Check sheet for the modelled part. Datum: model origin and axes. Units: mm. Round coordinates to 2 decimals unless told otherwise and drop trailing zeros. Order: outer loops, then holes, each group sorted by start corner. A loop starts at its lowest first (then second) coordinate and runs counter-clockwise, first axis right, second up. Notation, with made-up numbers: (-14, -8.5) -> (44, -8.5) arc R18 ccw to (44, 2.5) -> close; hole circle Ø1 at (67.5, 55.5). An arc over 180 degrees is marked (long way). Answer in a Markdown table with one row per item.
```python
from build123d import *

# Parameters (mm, degrees)
SKETCH_1_W          = 164
SKETCH_1_H          = 215
SKETCH_1_R          = 14.5
EXTRUDE_1_DEPTH     = 3
SKETCH_2_R          = 2
CUT_EXTRUDE_1_DEPTH = 3
SKETCH_3_W          = 3
SKETCH_3_H          = 25
CUT_EXTRUDE_2_DEPTH = 10
SKETCH_4_W          = 15
SKETCH_4_H          = 3
CUT_EXTRUDE_3_DEPTH = 10
SKETCH_6_W          = 10
SKETCH_6_H          = 190
EXTRUDE_2_DEPTH     = 3
CHAMFER_1_SIZE      = 25
CHAMFER_1_SIZE_2    = 14.43375673
FILLET_3_R          = 20
FILLET_4_R          = 10


with BuildPart() as part:
    # 草图1 → 凸台-拉伸1 (new body)
    with BuildSketch(Plane(origin=(0, 0, 0), x_dir=(1, 0, 0), z_dir=(0, 1, 0))):
        with Locations((47, 70)):
            Rectangle(SKETCH_1_W, SKETCH_1_H)
        with Locations(Location((94, 40, 0), (0, 0, 270))):
            Circle(SKETCH_1_R, mode=Mode.SUBTRACT)
        with Locations(Location((0, 40, 0), (0, 0, 270))):
            Circle(SKETCH_1_R, mode=Mode.SUBTRACT)
        with Locations(Location((0, 145, 0), (0, 0, 270))):
            Circle(SKETCH_1_R, mode=Mode.SUBTRACT)
        with Locations(Location((94, 145, 0), (0, 0, 270))):
            Circle(SKETCH_1_R, mode=Mode.SUBTRACT)
    extrude(amount=EXTRUDE_1_DEPTH)

    # 草图2 → 切除-拉伸1 (cut)
    with BuildSketch(Plane(origin=(0, 3, 0), x_dir=(1, 0, 0), z_dir=(0, 1, 0))):
        with Locations(Location((0, -27.5, 0), (0, 0, 270))):
            Circle(SKETCH_2_R)
        with Locations(Location((-15, -27.5, 0), (0, 0, 270))):
            Circle(SKETCH_2_R)
        with Locations(Location((15, -27.5, 0), (0, 0, 90))):
            Circle(SKETCH_2_R)
        with Locations(Location((79, -27.5, 0), (0, 0, 270))):
            Circle(SKETCH_2_R)
        with Locations(Location((109, -27.5, 0), (0, 0, 90))):
            Circle(SKETCH_2_R)
        with Locations(Location((94, -27.5, 0), (0, 0, 90))):
            Circle(SKETCH_2_R)
    extrude(amount=-CUT_EXTRUDE_1_DEPTH, mode=Mode.SUBTRACT)

    # 草图3 → 切除-拉伸2 (cut)
    with BuildSketch(Plane(origin=(0, 3, 0), x_dir=(1, 0, 0), z_dir=(0, 1, 0))):
        with Locations((28.5, 135)):
            Rectangle(SKETCH_3_W, SKETCH_3_H)
        with Locations((65.5, 135)):
            Rectangle(SKETCH_3_W, SKETCH_3_H)
        with Locations((28.5, 75)):
            Rectangle(SKETCH_3_W, SKETCH_3_H)
        with Locations((65.5, 75)):
            Rectangle(SKETCH_3_W, SKETCH_3_H)
        with Locations((28.5, 15)):
            Rectangle(SKETCH_3_W, SKETCH_3_H)
        with Locations((65.5, 15)):
            Rectangle(SKETCH_3_W, SKETCH_3_H)
        with Locations((-28.5, 15)):
            Rectangle(SKETCH_3_W, SKETCH_3_H)
        with Locations((-28.5, 75)):
            Rectangle(SKETCH_3_W, SKETCH_3_H)
        with Locations((-28.5, 135)):
            Rectangle(SKETCH_3_W, SKETCH_3_H)
        with Locations((122.5, 135)):
            Rectangle(SKETCH_3_W, SKETCH_3_H)
        with Locations((122.5, 75)):
            Rectangle(SKETCH_3_W, SKETCH_3_H)
        with Locations((122.5, 15)):
            Rectangle(SKETCH_3_W, SKETCH_3_H)
    extrude(amount=-CUT_EXTRUDE_2_DEPTH, mode=Mode.SUBTRACT)

    # 草图4 → 切除-拉伸3 (cut)
    with BuildSketch(Plane(origin=(0, 3, 0), x_dir=(1, 0, 0), z_dir=(0, 1, 0))):
        with Locations((-0.5, 170)):
            Rectangle(SKETCH_4_W, SKETCH_4_H)
        with Locations((94.5, 170)):
            Rectangle(SKETCH_4_W, SKETCH_4_H)
    extrude(amount=-CUT_EXTRUDE_3_DEPTH, mode=Mode.SUBTRACT)

    # 草图6 → 凸台-拉伸2 (add)
    with BuildSketch(Plane(origin=(0, 3, 0), x_dir=(1, 0, 0), z_dir=(0, 1, 0))):
        with Locations((-40, 82.5)):
            Rectangle(SKETCH_6_W, SKETCH_6_H)
        with Locations((134, 82.5)):
            Rectangle(SKETCH_6_W, SKETCH_6_H)
    extrude(amount=-EXTRUDE_2_DEPTH)

    # 倒角1
    # the kernel refuses this chamfer: 25, 14.43375673 mm, written as the material it takes off along each edge
    with BuildSketch(Plane(origin=(139, 67.677143866, 12.5), x_dir=(0.019326765612700705, 0, -0.9998132206222079), z_dir=(0, -1, 0))) as chamfer_1_piece_1_section:
        Polygon((CHAMFER_1_SIZE * 0.999813220622, -CHAMFER_1_SIZE * 0.0193267656127), (-CHAMFER_1_SIZE_2 * 0.0193267656124, -CHAMFER_1_SIZE_2 * 0.999813220604), (0, 0), align=None)
    chamfer_1_piece_1 = extrude(amount=132.354287732, mode=Mode.PRIVATE)
    chamfer_1_piece_1 = split(chamfer_1_piece_1, bisect_by=Plane(origin=(129, 1.5, 3.344472452), z_dir=(1, 0, 0)), keep=Keep.TOP, mode=Mode.PRIVATE)
    add(chamfer_1_piece_1, mode=Mode.SUBTRACT)
    with BuildSketch(Plane(origin=(-45, 67.677143866, 12.5), x_dir=(0.9983227437537926, 0, 0.057893862402670776), z_dir=(0, -1, 0))) as chamfer_1_piece_2_section:
        Polygon((CHAMFER_1_SIZE_2 * 0.998322743736, -CHAMFER_1_SIZE_2 * 0.0578938624016), (-CHAMFER_1_SIZE * 0.0578938624027, -CHAMFER_1_SIZE * 0.998322743754), (0, 0), align=None)
    chamfer_1_piece_2 = extrude(amount=132.354287732, mode=Mode.PRIVATE)
    chamfer_1_piece_2 = split(chamfer_1_piece_2, bisect_by=Plane(origin=(-35, 1.5, 3.344472452), z_dir=(-1, 0, 0)), keep=Keep.TOP, mode=Mode.PRIVATE)
    add(chamfer_1_piece_2, mode=Mode.SUBTRACT)

    # 圆角3
    fillet_3_edges = [part.edges().sort_by_distance(p)[0] for p in [
        (139, 1.5, -12.5),
        (-45, 1.5, -12.5),
        (129, 1.5, 4.820508076),
        (-35, 1.5, 4.820508076),
    ]]
    fillet(fillet_3_edges, radius=FILLET_3_R)

    # 圆角4
    fillet_4_edges = [part.edges().sort_by_distance(p)[0] for p in [
        (-35, 1.5, 37.5),
        (129, 1.5, 37.5),
        (-45, 1.5, -177.5),
        (139, 1.5, -177.5),
    ]]
    fillet(fillet_4_edges, radius=FILLET_4_R)


solid = part.part
```
(1) Section check A-A on z = -145. Record the boundary of the cut face in (x, y).
Solutions:
| item | result |
|---|---|
| outline | (-45, 0) -> (-30, 0) -> (-30, 3) -> (-45, 3) -> close; (-27, 0) -> (-14.5, 0) -> (-14.5, 3) -> (-27, 3) -> close; (14.5, 0) -> (27, 0) -> (27, 3) -> (14.5, 3) -> close; (30, 0) -> (64, 0) -> (64, 3) -> (30, 3) -> close; (67, 0) -> (79.5, 0) -> (79.5, 3) -> (67, 3) -> close; (108.5, 0) -> (121, 0) -> (121, 3) -> (108.5, 3) -> close; (124, 0) -> (139, 0) -> (139, 3) -> (124, 3) -> close |
(2) Depth check by flat-ended pin: pin 1 Ø4.5 at (x, z) = (109, 27.5) entering from +Y; pin 2 Ø0.9 at (x, y) = (-28, 2) entering from +Z; pin 3 Ø0.9 at (y, z) = (1, -15) entering from +X. Enter the tip coordinate at first touch or a pass-through.
Solutions:
| item | result |
|---|---|
| pin 1 | y = 3 |
| pin 2 | z = 37.17 |
| pin 3 | x = 138.85 |
(3) Draft check along X on faces 1 (the cylindrical face through (135.99, 1.48, -174.65)), 2 (the cylindrical face through (0.638, 1.479, -159.486)), 3 (the flat face through (46, 3, -72)). Enter one of: pulls with the +X half, pulls with the -X half, needs draft (parallel to the pull), parting line crosses it, or undercut.
Solutions:
| item | result |
|---|---|
| face 1 | pulls with the +X half |
| face 2 | undercut |
| face 3 | needs draft |
(4) Scan lines: probe 1 along X at (y, z) = (2.4, -71.5); probe 2 along Z at (x, y) = (15, 0.9); probe 3 along Z at (x, y) = (-3.5, 2.5). Record each from-to range of solid material in increasing order. Write a range as from..to.
Solutions:
| item | result |
|---|---|
| probe 1 | -45..-30, -27..27, 30..64, 67..121, 124..139 |
| probe 2 | -177.5..25.5, 29.5..37.5 |
| probe 3 | -177.5..-171.5, -168.5..-159.07, -130.93..-54.07, -25.93..37.5 |
(5) Section check B-B on z = -10.5. Record the boundary of the cut face in (x, y).
Solutions:
| item | result |
|---|---|
| outline | (-43.6, 0) -> (-30, 0) -> (-30, 3) -> (-43.6, 3) -> close; (-27, 0) -> (27, 0) -> (27, 3) -> (-27, 3) -> close; (30, 0) -> (64, 0) -> (64, 3) -> (30, 3) -> close; (67, 0) -> (121, 0) -> (121, 3) -> (67, 3) -> close; (124, 0) -> (137.6, 0) -> (137.6, 3) -> (124, 3) -> close |
(6) Section check C-C on y = 1.8. Give the number of separate pieces and of enclosed holes in the cut face, plus the area to 3 significant figures.
Solutions:
| item | result |
|---|---|
| separate pieces | 1 |
| enclosed holes | 24 |
| area | 34,900 mm^2 |
